from build123d import *

# Parameters (mm, degrees)
CUT_EXTRUDE_1_DEPTH    = 10.2
EXTRUDE_1_DEPTH        = 32
HOLE_WIZARD_M2_1_D     = 1.6
HOLE_WIZARD_M2_1_DEPTH = 5
HOLE_WIZARD_M2_1_TIP   = 0.480688495


with BuildPart() as part:
    # 草图1 → 旋转1 (revolve)
    with BuildSketch(Plane.XY, mode=Mode.PRIVATE) as revolve_1_sk:
        Polygon((0, 0), (11, 0), (11, 64.9), (10.5, 64.9), (10.5, 65.9), (11, 65.9), (11, 97.9), (7.5, 97.9), (7.5, 100), (3, 100), (3, 114.2), (0, 114.2), align=None)
    revolve(revolve_1_sk.sketch.rotate(Axis((0, 60.650671984, 0), (0, -1, 0)), 90), axis=Axis((0, 60.650671984, 0), (0, -1, 0)))

    # 草图2 → 切除-拉伸1 (cut)
    with BuildSketch(Plane(origin=(0, 114.2, 0), x_dir=(1, 0, 0), z_dir=(0, 1, 0))):
        Polygon((-48.862110032, 2.4), (-1.8, 2.4), (1.8, 2.4), (48.862110032, 2.4), (48.862110032, 96.524220063), (-48.862110032, 96.524220063), align=None)
    extrude(amount=-CUT_EXTRUDE_1_DEPTH, mode=Mode.SUBTRACT)

    # 草图3 → 凸台-拉伸1 (add)
    with BuildSketch(Plane.XZ):
        with BuildLine():
            Line((-16, 0), (-16, -35))
            ThreePointArc((-16, -35), (0, -42), (16, -35))
            Line((16, -35), (16, 0))
            ThreePointArc((16, 0), (0, 16), (-16, 0))
        make_face()
    extrude(amount=EXTRUDE_1_DEPTH)

    # M2 螺纹孔1
    with Locations(Plane(origin=(0, 97.9, 0), x_dir=(1, 0, 0), z_dir=(0, 1, 0))):
        with Locations((0, 9.5), (-8.227241336, 4.75), (-8.227241336, -4.75), (0, -9.5), (8.227241336, -4.75), (8.227241336, 4.75)):
            Hole(HOLE_WIZARD_M2_1_D / 2, depth=HOLE_WIZARD_M2_1_DEPTH)
            with Locations((0, 0, -(HOLE_WIZARD_M2_1_DEPTH + HOLE_WIZARD_M2_1_TIP / 2))):  # 118° drill point
                Cone(0, HOLE_WIZARD_M2_1_D / 2, HOLE_WIZARD_M2_1_TIP, mode=Mode.SUBTRACT)


solid = part.part
Here's how the part is built. I have some questions about the finished solid (model axes, mm). A direction names the side the tool comes from. Round coordinates to 2 decimals unless told otherwise and drop trailing zeros. Loops run counter-clockwise (first coordinate to the right, second up) from the corner with the lowest first, then second, coordinate; pieces in that order, holes last.
1. For P1, Ø6, axis at x = -8.5, y = 77.5, coming from the +Z side; P2, Ø6, axis at x = 9, z = -5, coming from the +Y side; P3, Ø1.4, axis at x = 8.23, z = -4.75, coming from the +Y side; P4, Ø11, axis at x = -3.5, z = -3, coming from the +Y side, each with a flat end and sliding along its axis, tell me the tip position at first contact or that it passes through.
Answer list:
P1: stops at z = 9.53
P2: stops at y = 100
P3: stops at y = 92.84
P4: stops at y = 114.2
2. If I drill on line 1 along X through (y, z) = (95.45, -9.5); line 2 along X through (y, z) = (95, -4.75); line 3 along Y through (x, z) = (10.5, -21), over which ranges is the centre line in solid material (lowest first)?
Answer list:
line 1: x = -5.55 to -0.8, 0.8 to 5.55
line 2: x = -9.92 to -9.03, -7.43 to 7.43, 9.03 to 9.92
line 3: y = -32 to 0
3. We'd pull the mould along Y, two halves only. Please class faces 1 (the face through (-3.2, 65.4, 10)), 2 (the face through (10.74, 32.9, -2.38)), 3 (the face through (0, 0, -19)): +Y half, -Y half, draft (parallel to the pull), parting line (faces both ways), or undercut.
Answer list:
face 1: undercut
face 2: draft
face 3: +Y half
4. If we section it at B-B on y = -15: Write out the boundary of the cut face in (x, z).
Answer list:
outline: (-16, -35) arc R21.79 ccw to (16, -35) - (16, 0) arc R16 ccw to (-16, 0) - close
5. Which directions (+Z, -Z, +X, -X, +Y, -Y) give clear straight access to the entire face, cutting with the end or side of a thin tool? Please do faces 4 (the face through (10, 65.9, -4)), 5 (the face through (10.74, 82.12, -2.38)), 6 (the face through (0, 109, -2.4)).
Answer list:
face 4: none
face 5: +Y
face 6: -Z, +X, -X, +Y
6. If we section it at A-A on z = -30: Write out the boundary of the cut face in (x, y).
Answer list:
outline: (-16, -32) - (16, -32) - (16, 0) - (-16, 0) - close
7. If we section it at C-C on y = 55.5: Write out the boundary of the cut face in (x, z).
Answer list:
outline: circle Ø22 at (0, 0)
